Verification items for the finished model (mm, model axes). A direction names the side the tool comes from. Coordinates: 2 decimals unless noted, no trailing zeros. Write each loop counter-clockwise with the first axis right and the second up, starting at its lowest first coordinate (ties: lowest second). Pieces come first, ordered by that corner, then holes. Notation, with made-up numbers: (82, 88) -> (90, 88) arc R23 cw to (90, 126) -> close; hole circle Ø9 at (40, 70.5). An arc over 180 degrees is marked (long way). Answer in a Markdown table with one row per item.
```python
from build123d import *

# Parameters (mm, degrees)
EXTRUDE_THIN1_DEPTH     = 25.4
SKETCH3_R               = 2.5
CUT_EXTRUDE1_DEPTH      = 10
CUT_EXTRUDE2_DEPTH      = 148.922817712
CUT_EXTRUDE2_DEPTH_BACK = 148.922817712
SKETCH4_R               = 2.5


with BuildPart() as part:
    # Sketch2 → Extrude-Thin1 (new body)
    with BuildSketch(Plane.XY):
        Polygon((-105, -100), (-105, -75), (-40, 0), (40, 0), (105, -75), (105, -100), (106, -100), (106, -74.626966674), (40.456628883, 1), (-40.456628883, 1), (-106, -74.626966674), (-106, -100), align=None)
    extrude(amount=EXTRUDE_THIN1_DEPTH)

    # Sketch3 → Cut-Extrude1 (cut)
    with BuildSketch(Plane(origin=(0, 1, 0), x_dir=(1, 0, 0), z_dir=(0, 1, 0))):
        with Locations(Location((-25, -12.7, 0), (0, 0, 270))):
            Circle(SKETCH3_R)
        with Locations(Location((25, -12.7, 0), (0, 0, 270))):
            Circle(SKETCH3_R)
    extrude(amount=-CUT_EXTRUDE1_DEPTH, mode=Mode.SUBTRACT)

    # Sketch4 → Cut-Extrude2 (cut, two sides: drawn at the far end of the back side and taken through both)
    with BuildSketch(Plane(origin=(0, 0, 0), x_dir=(0, 0, -1), z_dir=(1, 0, 0)).offset(-CUT_EXTRUDE2_DEPTH_BACK)):
        with Locations((-12.7, -87.313483337)):
            Circle(SKETCH4_R)
    extrude(amount=CUT_EXTRUDE2_DEPTH + CUT_EXTRUDE2_DEPTH_BACK, mode=Mode.SUBTRACT)


solid = part.part
```
1. Material ranges on probe 1 along X at (y, z) = (-89, 23.25); probe 2 along X at (y, z) = (0.8, 12.7); probe 3 along Y at (x, z) = (-1, 10.25), recorded low to high. Write a range as from..to.
Findings below:
| item | result |
|---|---|
| probe 1 | x = -106..-105, 105..106 |
| probe 2 | x = -40.63..-27.5, -22.5..22.5, 27.5..40.63 |
| probe 3 | y = 0..1 |
2. Access from +Z, -Z, +X, -X, +Y, -Y to the whole of each face (thin tool, end or side, straight path). Record for faces 1 (the face through (1, 1, 13)), 2 (the face through (-72.95, -38.02, 12.52)).
Findings below:
| item | result |
|---|---|
| face 1 | +Z, -Z, +X, -X, +Y |
| face 2 | +Z, -Z, -Y |
3. Sectioned sample at D-D, the plane y = -20. Record the cut outline in (x, z).
Findings below:
| item | result |
|---|---|
| outline | (-58.66, 0) -> (-57.33, 0) -> (-57.33, 25.4) -> (-58.66, 25.4) -> close; (57.33, 0) -> (58.66, 0) -> (58.66, 25.4) -> (57.33, 25.4) -> close |
4. Sectioned sample at C-C, the plane z = 23.25. Record the cut outline in (x, y), and give its area (3 significant figures).
Findings below:
| item | result |
|---|---|
| outline | (-106, -100) -> (-105, -100) -> (-105, -75) -> (-40, 0) -> (40, 0) -> (105, -75) -> (105, -100) -> (106, -100) -> (106, -74.63) -> (40.46, 1) -> (-40.46, 1) -> (-106, -74.63) -> close |
| area | 330 mm² |
5. Sectioned sample at B-B, the plane z = 12.7. Record the cut outline in (x, y).
Findings below:
| item | result |
|---|---|
| outline | (-106, -100) -> (-105, -100) -> (-105, -89.81) -> (-106, -89.81) -> close; (-106, -84.81) -> (-105, -84.81) -> (-105, -75) -> (-40, 0) -> (-27.5, 0) -> (-27.5, 1) -> (-40.46, 1) -> (-106, -74.63) -> close; (-22.5, 0) -> (22.5, 0) -> (22.5, 1) -> (-22.5, 1) -> close; (27.5, 0) -> (40, 0) -> (105, -75) -> (105, -84.81) -> (106, -84.81) -> (106, -74.63) -> (40.46, 1) -> (27.5, 1) -> close; (105, -100) -> (106, -100) -> (106, -89.81) -> (105, -89.81) -> close |
6. Go/stop test with flat-tipped pins: pin 1 (3 mm diameter, centred on y = -87.31, z = 12.7, fed in from +X); pin 2 (8 mm diameter, centred on y = -74, z = 9, fed in from +X); pin 3 (10 mm diameter, centred on y = -53, z = 18, fed in from +X); pin 4 (1.5 mm diameter, centred on x = -52, z = 5, fed in from -Y). Record where each tip stops, or that it passes through.
Findings below:
| item | result |
|---|---|
| pin 1 | passes through |
| pin 2 | stops at x = 106 |
| pin 3 | stops at x = 91.59 |
| pin 4 | stops at y = -14.71 |
7. Release check for a two-part mould opening along Z. For faces 3 (the face through (105, -90, 13)), 4 (the face through (-105.507, -84.835, 13.025)) record: released by +Z, released by -Z, zero draft, split by the parting line, or undercut.
Findings below:
| item | result |
|---|---|
| face 3 | zero draft |
| face 4 | undercut |
8. Sectioned sample at A-A, the plane x = -25. Record the cut outline in (y, z), and give its area (3 significant figures).
Findings below:
| item | result |
|---|---|
| outline | (0, 0) -> (1, 0) -> (1, 10.2) -> (0, 10.2) -> close; (0, 15.2) -> (1, 15.2) -> (1, 25.4) -> (0, 25.4) -> close |
| area | 20.4 mm² |
